```python
from build123d import *

# Parameters (mm, degrees)
EXTRUDE_1_DEPTH = 3.5
SKETCH_2_R      = 2.5
EXTRUDE_2_DEPTH = 10


# Read off the part's stored shape, not the designer's step: M4x0.7 Машинная резьба Шпилька1
with BuildPart() as part:
    # Эскиз1 → Бобышка-Вытянуть1 (new body)
    with BuildSketch(Plane(origin=(0, 0, 0), x_dir=(1, 0, 0), z_dir=(0, 1, 0))):
        Polygon((1.309524818, -4.42927512), (4.490627183, -1.080555801), (3.181102365, 3.348719319), (-1.309524818, 4.42927512), (-4.490627183, 1.080555801), (-3.181102365, -3.348719319), align=None)
    extrude(amount=EXTRUDE_1_DEPTH)

    # Эскиз2 → Бобышка-Вытянуть2 (add)
    with BuildSketch(Plane(origin=(0, 3.5, 0), x_dir=(1, 0, 0), z_dir=(0, 1, 0))):
        with Locations(Location((0, 0, 0), (0, 0, 270))):
            Circle(SKETCH_2_R)
    extrude(amount=EXTRUDE_2_DEPTH)

    # M4x0.7 Машинная резьба Шпилька1 outline → M4x0.7 Машинная резьба Шпилька1 (revolve, cut)
    with BuildSketch(Plane.XY):
        Polygon((2, 13.11), (2, 3.5), (2.5, 3.5), (2.5, 13.5), (1.61, 13.5), align=None)
    revolve(axis=Axis((0, 0, 0), (0, 1, 0)), mode=Mode.SUBTRACT)


solid = part.part
```
Part model, mm, in its own coordinate system. A direction names the side the tool comes from. Coordinates: 2 decimals unless noted, no trailing zeros. Order: outer loops, then holes, each group sorted by start corner. A loop starts at its lowest first (then second) coordinate and runs counter-clockwise, first axis right, second up. Notation, with made-up numbers: (77, -7.75) -> (128, -7.75) arc R16 ccw to (128, 3.25) -> close; hole circle Ø1 at (23.25, 9). An arc over 180 degrees is marked (long way). Put each result on its own line as item: value. Start each with the question number.
(1) Band-saw the part on B-B (z = 0). Give the cut face in (x, y), then the cut area to 3 significant figures.
(2) Probe line 1 along Y through (x, z) = (2, 1.25); line 2 along X through (y, z) = (9.25, 0); line 3 along Z through (x, y) = (2, 3.25). List the from-to ranges inside material, lowest first. Write a range as [from, to].
(3) Band-saw the part on D-D (y = 9.75). Give the cut face in (x, z).
(4) Which spindle directions (+Z, -Z, +X, -X, +Y, -Y) get a long thin tool onto all of the face, cutting with end or side? Do faces 1 (the face through (-3.845, 1.726, 1.103)), 2 (the face through (-1, 3.5, -2)). Say none if no direction does.
(5) Band-saw the part on A-A (y = 2.5). Give the cut face in (x, z), then the cut area to 3 significant figures.
(6) Pin check, flat tips, straight feed: pin 1 Ø2 at (x, y) = (-1, 12) entering from +Z; pin 2 Ø2 at (x, y) = (-1.5, 5.5) entering from -Z. Stop position of each tip, or through.
(7) Band-saw the part on C-C (x = 0). Give the cut face in (y, z), then the cut area to 3 significant figures.
Determined:
1. outline: (-4.17, 0) -> (4.17, 0) -> (4.17, 3.5) -> (2, 3.5) -> (2, 13.11) -> (1.61, 13.5) -> (-1.61, 13.5) -> (-2, 13.11) -> (-2, 3.5) -> (-4.17, 3.5) -> close
1. area: 69.0 mm²
2. line 1: y = [0, 3.5]
2. line 2: x = [-2, 2]
2. line 3: z = [-3.63, 3.7]
3. outline: circle Ø4 at (0, 0)
4. face 1: +Z, -X, +Y, -Y
4. face 2: +Y
5. outline: (-4.49, -1.08) -> (-1.31, -4.43) -> (3.18, -3.35) -> (4.49, 1.08) -> (1.31, 4.43) -> (-3.18, 3.35) -> close
5. area: 55.4 mm²
6. pin 1: stops at z = 2
6. pin 2: stops at z = -1.94
7. outline: (0, -4.11) -> (3.5, -4.11) -> (3.5, -2) -> (13.11, -2) -> (13.5, -1.61) -> (13.5, 1.61) -> (13.11, 2) -> (3.5, 2) -> (3.5, 4.11) -> (0, 4.11) -> close
7. area: 68.6 mm²
